Work out the finished part from the listing and answer in its coordinate system (mm). Face numbers are marked on the shaded views. A direction names the side the tool comes from. Coordinates: 2 decimals unless noted, no trailing zeros. Loops run counter-clockwise (first coordinate to the right, second up) from the corner with the lowest first, then second, coordinate; pieces in that order, holes last. Notation, with made-up numbers: (42, 88.5) -> (65, 88.5) arc R31 cw to (65, 125.5) -> close; hole circle Ø1 at (62.5, -18). An arc over 180 degrees is marked (long way). Answer as CSV lines item,"result".
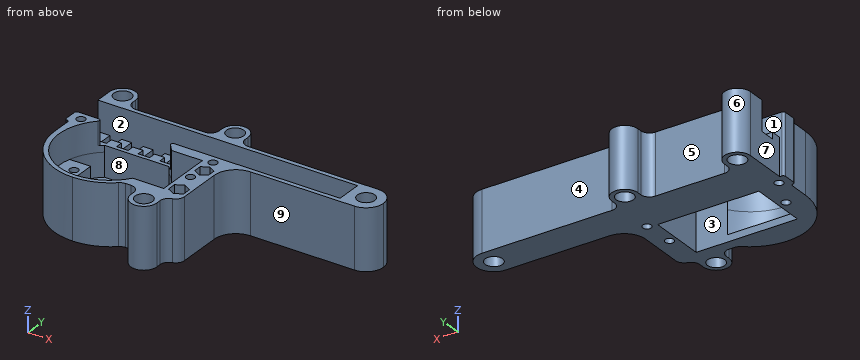
```python
from build123d import *

# Parameters (mm, degrees)
BODY_DEPTH                      = 14
HAUPTAUSTRAGUNG_DEPTH           = 6.9
SERVOSCHNITT_DEPTH              = 69.010587411
SERVOSCHNITT_DEPTH_BACK         = 69.010587411
SERVO_W                         = 23.4
SERVO_H                         = 13.2
VERRUNDUNG2_R                   = 5
SCHRAUBENLOCH_DEPTH             = 69.010587411
SCHRAUBENLOCH_DEPTH_BACK        = 69.010587411
SERVOLOCHSCHRAUBEN_R            = 1
FUEHRUNG_W                      = 60
FUEHRUNG_H                      = 2.5
FUEHRUNGSSCHINE_DEPTH           = 1.5
VERRUNDUNG4_R                   = 2
HALTERUNG_R                     = 1
SCHNITT_LINEAR_AUSTRAGEN2_DEPTH = 69.010587411
SKIZZE5_R                       = 1
SCHNITT_LINEAR_AUSTRAGEN3_DEPTH = 69.010587411
SCHNITT_LINEAR_START            = -6
SKIZZE8_W                       = 2.673131507
SKIZZE8_H                       = 5.13849065
SCHNITT_LINEAR_AUSTRAGEN7_DEPTH = 73.931681587
LINEARES_MUSTER1_COUNT          = 11
LINEARES_MUSTER1_PITCH          = 5
SABSCHLUSS_W                    = 8
SABSCHLUSS_H                    = 8
ABSCHLUSS_DEPTH                 = 14
SKIZZE14_R                      = 2
ENDSTUTZEN_DEPTH                = 14
SKIZZESTUTZEN_R                 = 2
STUTZEN_DEPTH                   = 14
VERRUNDUNG5_R                   = 4
VERRUNDUNG6_R                   = 2
VERRUNDUNG7_R                   = 2
SECHSKANTLOCH_DEPTH             = 13
HALTERUNGLINKS_DEPTH            = 5.5
SKIZZE15_R                      = 2
AUFSATZ_LINEAR_AUSTRAGEN1_DEPTH = 14
VERRUNDUNG8_R                   = 2
SKIZZE16_W                      = 1
SKIZZE16_H                      = 3.8
AUFSATZ_LINEAR_AUSTRAGEN2_DEPTH = 14
VERRUNDUNG10_R                  = 0.5
VERRUNDUNG11_R                  = 0.5
VERRUNDUNG12_R                  = 0.5


with BuildPart() as part:
    # P-BodySkizze → body (new body)
    with BuildSketch(Plane.XY):
        with BuildLine():
            Line((0, 0), (60, 0))
            Line((60, 0), (60, -8))
            Line((60, -8), (35, -8))
            Line((35, -8), (35, -25.18083152))
            Line((35, -25.18083152), (22, -25.18083152))
            ThreePointArc((22, -25.18083152), (17.850215987, -27.861318538), (13, -28.8))
            ThreePointArc((13, -28.8), (3.807611845, -24.992388155), (0, -15.8))
            Line((0, -15.8), (0, 0))
        make_face()
    extrude(amount=BODY_DEPTH)

    # Austrag → hauptAustragung (cut)
    with BuildSketch(Plane.XY.offset(14)):
        with BuildLine():
            ThreePointArc((20.443697295, -7), (13.002720829, -4.343644442), (5.561744363, -7))
            Line((5.561744363, -7), (20.443697295, -7))
        make_face()
        with BuildLine():
            Line((20.443697295, -7), (5.561744363, -7))
            ThreePointArc((5.561744363, -7), (7.971268428, -26.711882843), (24.752720829, -16.093644442))
            ThreePointArc((24.752720829, -16.093644442), (23.62095923, -11.062192041), (20.443697295, -7))
        make_face()
        with BuildLine():
            Line((60, -1), (0, -1))
            Line((0, -1), (0, -7))
            Line((0, -7), (5.561744363, -7))
            ThreePointArc((5.561744363, -7), (13.002720829, -4.343644442), (20.443697295, -7))
            Line((20.443697295, -7), (60, -7))
            Line((60, -7), (60, -1))
        make_face()
    extrude(amount=-HAUPTAUSTRAGUNG_DEPTH, mode=Mode.SUBTRACT)

    # servo → ServoSchnitt (cut, two sides: drawn at the far end of the back side and taken through both)
    with BuildSketch(Plane.XY.offset(14).offset(-SERVOSCHNITT_DEPTH_BACK)):
        with Locations((18.202720829, -16.093644442)):
            Rectangle(SERVO_W, SERVO_H)
    extrude(amount=SERVOSCHNITT_DEPTH + SERVOSCHNITT_DEPTH_BACK, mode=Mode.SUBTRACT)

    # Verrundung2
    verrundung2_edges = [part.edges().sort_by_distance(p)[0] for p in [
        (35, -8, 7),
    ]]
    fillet(verrundung2_edges, radius=VERRUNDUNG2_R)

    # servolochschrauben → schraubenloch (cut, two sides: drawn at the far end of the back side and taken through both)
    with BuildSketch(Plane.XY.offset(14).offset(-SCHRAUBENLOCH_DEPTH_BACK)):
        with Locations((4.702720829, -16.094776923)):
            Circle(SERVOLOCHSCHRAUBEN_R)
        with Locations((31.602720829, -16.094776923)):
            Circle(SERVOLOCHSCHRAUBEN_R)
    extrude(amount=SCHRAUBENLOCH_DEPTH + SCHRAUBENLOCH_DEPTH_BACK, mode=Mode.SUBTRACT)

    # fuehrung → Fuehrungsschine (add)
    with BuildSketch(Plane.XY.offset(7.1)):
        with Locations((30, -5.75)):
            Rectangle(FUEHRUNG_W, FUEHRUNG_H)
    extrude(amount=FUEHRUNGSSCHINE_DEPTH)

    # Verrundung4
    verrundung4_edges = [part.edges().sort_by_distance(p)[0] for p in [
        (35, -25.18083152, 7),
    ]]
    fillet(verrundung4_edges, radius=VERRUNDUNG4_R)

    # halterung → Schnitt-Linear austragen2 (cut, through all)
    with BuildSketch(Plane.XY.offset(14)):
        with Locations((1.5, -9)):
            Circle(HALTERUNG_R)
    extrude(amount=-SCHNITT_LINEAR_AUSTRAGEN2_DEPTH, mode=Mode.SUBTRACT)

    # Skizze5 → Schnitt-Linear austragen3 (cut, through all)
    with BuildSketch(Plane.XY.offset(14)):
        with Locations((32, -9)):
            Circle(SKIZZE5_R)
    extrude(amount=-SCHNITT_LINEAR_AUSTRAGEN3_DEPTH, mode=Mode.SUBTRACT)

    # Skizze8 → Schnitt-Linear austragen7 (cut)
    with BuildSketch(Plane.XY.offset(7.1).offset(SCHNITT_LINEAR_START)):
        with Locations((4.124861588, -3.569245325)):
            Rectangle(SKIZZE8_W, SKIZZE8_H)
    schnitt_linear_austragen7 = extrude(amount=SCHNITT_LINEAR_AUSTRAGEN7_DEPTH, mode=Mode.SUBTRACT)

    # Lineares Muster1: Schnitt-Linear austragen7 ×11
    with Locations(*[(i * LINEARES_MUSTER1_PITCH, 0, 0) for i in range(1, LINEARES_MUSTER1_COUNT)]):
        add(schnitt_linear_austragen7, mode=Mode.SUBTRACT)

    # sabschluss → Abschluss (add)
    with BuildSketch(Plane.XY.offset(14)):
        with Locations((64, -4)):
            Rectangle(SABSCHLUSS_W, SABSCHLUSS_H)
    extrude(amount=-ABSCHLUSS_DEPTH)

    # Skizze14 → endstutzen (cut)
    with BuildSketch(Plane.XY.offset(14)):
        with Locations((64, -4)):
            Circle(SKIZZE14_R)
    extrude(amount=-ENDSTUTZEN_DEPTH, mode=Mode.SUBTRACT)

    # SkizzeStutzen → stutzen (add)
    # profile 1 of 2: a face of its own
    with BuildSketch(Plane.XY.offset(14)):
        with BuildLine():
            Line((32, -25.18083152), (26, -25.18083152))
            Line((26, -25.18083152), (26, -28.18083152))
            ThreePointArc((26, -28.18083152), (29, -31.18083152), (32, -28.18083152))
            Line((32, -28.18083152), (32, -25.18083152))
        make_face()
        with Locations((29, -28.18083152)):
            Circle(SKIZZESTUTZEN_R, mode=Mode.SUBTRACT)
    # profile 2 of 2: a face of its own
    with BuildSketch(Plane.XY.offset(14)):
        with BuildLine():
            Line((26, 3), (26, 0))
            Line((26, 0), (32, 0))
            Line((32, 0), (32, 3))
            ThreePointArc((32, 3), (29, 6), (26, 3))
        make_face()
        with Locations((29, 3)):
            Circle(SKIZZESTUTZEN_R, mode=Mode.SUBTRACT)
    extrude(amount=-STUTZEN_DEPTH)

    # Verrundung5
    verrundung5_edges = [part.edges().sort_by_distance(p)[0] for p in [
        (68, 0, 7),
        (68, -8, 7),
    ]]
    fillet(verrundung5_edges, radius=VERRUNDUNG5_R - 0.0001)  # a hair under: the kernel refuses the full size

    # Verrundung6
    verrundung6_edges = [part.edges().sort_by_distance(p)[0] for p in [
        (33, -25.18083152, 7),
        (26, -25.18083152, 7),
        (32, -25.18083152, 7),
        (32, 0, 7),
        (26, 0, 7),
    ]]
    fillet(verrundung6_edges, radius=VERRUNDUNG6_R)

    # Verrundung7
    verrundung7_edges = [part.edges().sort_by_distance(p)[0] for p in [
        (22, -25.18083152, 7),
    ]]
    fillet(verrundung7_edges, radius=VERRUNDUNG7_R)

    # sechskant-loch → sechskantloch (cut)
    with BuildSketch(Plane.XY.offset(14)):
        Polygon((34.261205516, -22.328313106), (34.238574988, -20.307713889), (32.477369472, -19.317012893), (30.738794484, -20.346911113), (30.761425012, -22.367510329), (32.522630528, -23.358211326), align=None)
        Polygon((32.465163938, -14.469262536), (34.059281734, -13.548898198), (34.059281734, -11.708169521), (32.465163938, -10.787805182), (30.871046143, -11.708169521), (30.871046143, -13.548898198), align=None)
    extrude(amount=-SECHSKANTLOCH_DEPTH, mode=Mode.SUBTRACT)

    # halterung links → halterungLinks (cut)
    with BuildSketch(Plane.XY.offset(7.1)):
        with BuildLine():
            Line((20.443697295, -7), (5.561744363, -7))
            ThreePointArc((5.561744363, -7), (3.120742136, -9.736837295), (1.642350763, -13.092895876))
            Line((1.642350763, -13.092895876), (6.502720829, -13.092895876))
            Line((6.502720829, -13.092895876), (6.502720829, -9.493644442))
            Line((6.502720829, -9.493644442), (22.723960462, -9.493644442))
            ThreePointArc((22.723960462, -9.493644442), (21.673936488, -8.164425124), (20.443697295, -7))
        make_face()
        with BuildLine():
            Line((6.502720829, -19.421283459), (1.733767081, -19.421283459))
            ThreePointArc((1.733767081, -19.421283459), (11.192764657, -27.703405794), (22.723960462, -22.693644442))
            Line((22.723960462, -22.693644442), (6.502720829, -22.693644442))
            Line((6.502720829, -22.693644442), (6.502720829, -19.421283459))
        make_face()
    extrude(amount=-HALTERUNGLINKS_DEPTH, mode=Mode.SUBTRACT)

    # Skizze15 → Aufsatz-Linear austragen1 (add)
    with BuildSketch(Plane.XY.offset(14)):
        with BuildLine():
            Line((0, 0), (6, 0))
            Line((6, 0), (6, 3))
            ThreePointArc((6, 3), (3, 6), (0, 3))
            Line((0, 3), (0, 0))
        make_face()
        with Locations((3, 3)):
            Circle(SKIZZE15_R, mode=Mode.SUBTRACT)
    extrude(amount=-AUFSATZ_LINEAR_AUSTRAGEN1_DEPTH)

    # Verrundung8
    verrundung8_edges = [part.edges().sort_by_distance(p)[0] for p in [
        (6, 0, 7),
    ]]
    fillet(verrundung8_edges, radius=VERRUNDUNG8_R)

    # Skizze16 → Aufsatz-Linear austragen2 (add)
    with BuildSketch(Plane.XY.offset(14)):
        with Locations((-0.5, -8.9)):
            Rectangle(SKIZZE16_W, SKIZZE16_H)
    extrude(amount=-AUFSATZ_LINEAR_AUSTRAGEN2_DEPTH)

    # Verrundung10
    verrundung10_edges = [part.edges().sort_by_distance(p)[0] for p in [
        (0, -10.8, 7),
        (-1, -10.8, 7),
        (-1, -7, 7),
    ]]
    fillet(verrundung10_edges, radius=VERRUNDUNG10_R - 0.0001)  # a hair under: the kernel refuses the full size

    # Verrundung11
    verrundung11_edges = [part.edges().sort_by_distance(p)[0] for p in [
        (5.561744363, -7, 11.3),
    ]]
    fillet(verrundung11_edges, radius=VERRUNDUNG11_R)

    # Verrundung12
    verrundung12_edges = [part.edges().sort_by_distance(p)[0] for p in [
        (20.443697295, -7, 11.3),
    ]]
    fillet(verrundung12_edges, radius=VERRUNDUNG12_R)


solid = part.part
```
(1) For a pull along X with two mould halves and no side action, classify the marked faces 6, 7, 8 and 9 as pulls with the +X half, pulls with the -X half, needs draft (parallel to the pull), parting line crosses it, or undercut.
Computed values:
face 6,"undercut"
face 7,"pulls with the -X half"
face 8,"undercut"
face 9,"needs draft"
(2) A cutting plane is placed at B-B, the plane x = 48.5. Write down the section's boundary in (y, z).
Computed values:
outline,"(-8, 0) -> (0, 0) -> (0, 14) -> (-1, 14) -> (-1, 1.1) -> (-6.14, 1.1) -> (-6.14, 8.6) -> (-7, 8.6) -> (-7, 14) -> (-8, 14) -> close"
(3) Consider line 1 along Y through (x, z) = (29, 5.25); line 2 along X through (y, z) = (-15.5, 7.5); line 3 along X through (y, z) = (-26, 12.75). Determine where each line is inside the solid, lowest interval first.
Computed values:
line 1,"-31.18 to -30.18, -26.18 to -22.69, -9.49 to -6.14, -1 to 1, 5 to 6"
line 2,"0 to 1.27, 29.9 to 30.8, 32.41 to 35"
line 3,"4.94 to 6.68, 19.32 to 21.06, 25.61 to 32.3"
(4) A cutting plane is placed at C-C, the plane x = 41.5. Write down the section's boundary in (y, z).
Computed values:
outline,"(-8, 0) -> (0, 0) -> (0, 14) -> (-1, 14) -> (-1, 7.1) -> (-4.5, 7.1) -> (-4.5, 8.6) -> (-7, 8.6) -> (-7, 14) -> (-8, 14) -> close"
(5) A cutting plane is placed at A-A, the plane y = -21. Write down the section's boundary in (x, z), and give its area (3 significant figures).
Computed values:
outline,"(1.09, 0) -> (6.5, 0) -> (6.5, 1.6) -> (2.33, 1.6) -> (2.33, 14) -> (1.09, 14) -> close; (29.9, 0) -> (35, 0) -> (35, 14) -> (34.25, 14) -> (34.25, 1) -> (30.75, 1) -> (30.75, 14) -> (29.9, 14) -> close"
area,"49.9 mm2"
(6) Flat-ended cylindrical pins translate along their axes: pin 1 Ø4 at (x, z) = (53, 5) entering from +Y; pin 2 Ø2.5 at (y, z) = (-4.5, 4) entering from -X; pin 3 Ø1.5 at (y, z) = (-27, 6.5) entering from -X. Find the tip coordinate at first contact, or state that the pin passes through.
Computed values:
pin 1,"y = 0"
pin 2,"x = 0"
pin 3,"x = 5.27"
(7) Which of the six approach directions +Z, -Z, +X, -X, +Y, -Y give full straight-line access (tool end or side, diameter ignored) to the marked faces 1, 2, 3, 4 and 5?
Computed values:
face 1,"+Z, -X"
face 2,"+Z"
face 3,"+Z, -Z"
face 4,"+Z, -Z, +X, +Y"
face 5,"+Z, -Z, +Y"
(8) A cutting plane is placed at D-D, the plane z = 3.25. Count the separate pieces of the cut face and the enclosed holes in it, and give its area (3 significant figures).
Computed values:
separate pieces,"1"
enclosed holes,"22"
area,"596 mm2"
